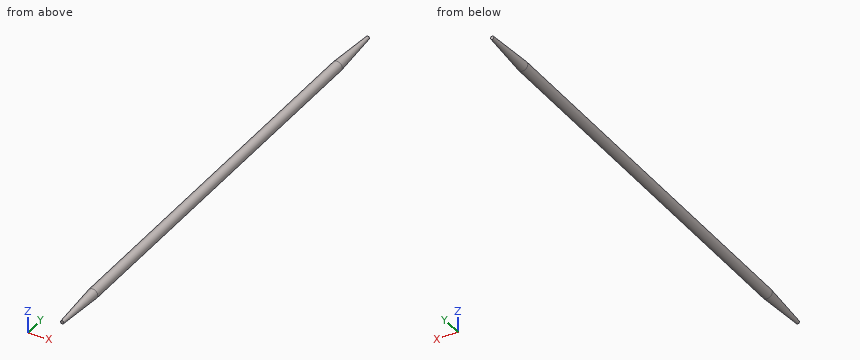
```python
from build123d import *

# Parameters (mm, degrees)
ESQUISSE1_R             = 1.5
BOSS_EXTRU_1_DEPTH      = 150
CHANFREIN1_SIZE         = 1
CHANFREIN1_SIZE2        = 15
CHANFREIN1_PART_2_SIZE  = 1
CHANFREIN1_PART_2_SIZE2 = 15


with BuildPart() as part:
    # Esquisse1 → Boss.-Extru.1 (new body)
    with BuildSketch(Plane(origin=(0, 0, 0), x_dir=(1, 0, 0), z_dir=(0, 1, 0))):
        Circle(ESQUISSE1_R)
    extrude(amount=BOSS_EXTRU_1_DEPTH)

    # Chanfrein1
    chanfrein1_edges = [part.edges().sort_by_distance(p)[0] for p in [
        (-1.5, 0, 0),
    ]]
    chanfrein1_side = [part.faces().sort_by_distance(p)[0] for p in [
        (0, 0, 0),
    ]]
    chamfer(chanfrein1_edges, length=CHANFREIN1_SIZE, length2=CHANFREIN1_SIZE2, reference=chanfrein1_side[0])

    # Chanfrein1 part 2
    chanfrein1_part_2_edges = [part.edges().sort_by_distance(p)[0] for p in [
        (-1.5, 150, 0),
    ]]
    chanfrein1_part_2_side = [part.faces().sort_by_distance(p)[0] for p in [
        (0, 150, 0),
    ]]
    chamfer(chanfrein1_part_2_edges, length=CHANFREIN1_PART_2_SIZE, length2=CHANFREIN1_PART_2_SIZE2, reference=chanfrein1_part_2_side[0])


solid = part.part
```
CAD build for the part. Positions are in the model's coordinates, mm. Round coordinates to 2 decimals unless told otherwise and drop trailing zeros. Loops run counter-clockwise (first coordinate to the right, second up) from the corner with the lowest first, then second, coordinate; pieces in that order, holes last. Notation, with made-up numbers: M 17.5,87.25 L 46.5,87.25 A11 ccw 46.5,107.25 Z; hole C 26,73 d5. An arc over 180 degrees is marked long. Use a Markdown table: item, result. Add a question column.
(1) Cut at D-D (y = 138). Give the cut face in (x, z).
(2) Drill centre lines: line 1 (X direction, y = 62, z = 0.3); line 2 (Z direction, x = -0.1, y = 113.5); line 3 (Z direction, x = -0.7, y = 105). Where is each one in solid material? Low to high.
(3) Cut at C-C (y = 16.5). Give the cut face in (x, z), and give its area (3 significant figures).
(4) Flat gauge pins, fed straight in: pin 1 (1 mm diameter, centred on y = 25, z = -1, fed in from +X); pin 2 (1 mm diameter, centred on x = 0.5, z = -0.5, fed in from +Y). Where does each tip first touch, or does it go through?
(5) Cut at B-B (z = 0). Give the cut face in (x, y), and give its area (3 significant figures).
(6) Cut at A-A (x = 0). Give the cut face in (y, z), and give its area (3 significant figures).
Geometry says:
| question | item | result |
|---|---|---|
| 1 | outline | C 0,0 d2.6 |
| 2 | line 1 | x = -1.47 to 1.47 |
| 2 | line 2 | z = -1.5 to 1.5 |
| 2 | line 3 | z = -1.33 to 1.33 |
| 3 | outline | C 0,0 d3 |
| 3 | area | 7.07 mm² |
| 4 | pin 1 | stops at x = 1.41 |
| 4 | pin 2 | stops at y = 150 |
| 5 | outline | M -1.5,15 L -0.5,0 L 0.5,0 L 1.5,15 L 1.5,135 L 0.5,150 L -0.5,150 L -1.5,135 Z |
| 5 | area | 420 mm² |
| 6 | outline | M 0,-0.5 L 15,-1.5 L 135,-1.5 L 150,-0.5 L 150,0.5 L 135,1.5 L 15,1.5 L 0,0.5 Z |
| 6 | area | 420 mm² |
